Can you work these out from the model? Positions are in its coordinate system, mm. Face numbers are marked on the shaded views. A direction names the side the tool comes from. Coordinates: 2 decimals unless noted, no trailing zeros. Write each loop counter-clockwise with the first axis right and the second up, starting at its lowest first coordinate (ties: lowest second). Pieces come first, ordered by that corner, then holes. Notation, with made-up numbers: (-1.75, -40) -> (4.25, -40) arc R5 ccw to (4.25, -36) -> close; hole circle Ø10 at (-29, 60). An arc over 180 degrees is marked (long way). Use one line per item in the form item = value.
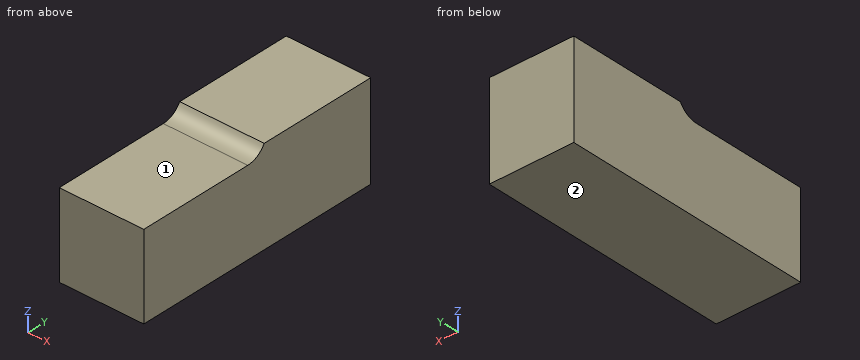
```python
from build123d import *

# Parameters (mm, degrees)
BOSS_EXTRUDE1_DEPTH = 25.4


with BuildPart() as part:
    # Sketch1 → Boss-Extrude1 (new body)
    with BuildSketch(Plane.YZ):
        with BuildLine():
            Line((0, 0), (76.2, 0))
            Line((76.2, 0), (76.2, 28.575))
            Line((76.2, 28.575), (40.424261314, 28.575))
            ThreePointArc((40.424261314, 28.575), (38.1, 26.250738686), (34.925, 25.4))
            Line((34.925, 25.4), (0, 25.4))
            Line((0, 25.4), (0, 0))
        make_face()
    extrude(amount=BOSS_EXTRUDE1_DEPTH)


solid = part.part
```
Q1. If I drill on line 1 (Z direction, x = 21.25, y = 27); line 2 (Z direction, x = 24, y = 39); line 3 (Y direction, x = 14.5, z = 26), over which ranges is the centre line in solid material (lowest first)? Write a range as from..to.
Return value:
line_1 = 0..25.4
line_2 = 0..26.88
line_3 = 37.62..76.2
Q2. Will these pins go through, and if not, where does the flat tip stop? pin 1 (2 mm diameter, centred on y = 59, z = 20.5, fed in from -X); pin 2 (5 mm diameter, centred on x = 14, y = 17, fed in from +Z).
Return value:
pin_1 = 0
pin_2 = 25.4
Q3. For the marked faces 1 and 2, which set-ups out of +Z, -Z, +X, -X, +Y, -Y let a thin tool reach every point of the face, with its end or its side?
Return value:
face_1 = +Z, +X, -X, -Y
face_2 = -Z, +X, -X, +Y, -Y
Q4. Suppose I cut it at A-A (x = 12). Write out the boundary of the cut face in (y, z) (3 decimals).
Return value:
outline = (0, 0) -> (76.2, 0) -> (76.2, 28.575) -> (40.424, 28.575) arc R6.35 cw to (34.925, 25.4) -> (0, 25.4) -> close
Q5. Suppose I cut it at B-B (y = 10.5). Write out the boundary of the cut face in (x, z).
Return value:
outline = (0, 0) -> (25.4, 0) -> (25.4, 25.4) -> (0, 25.4) -> close
